Could you check a few things on this model? Use its own coordinates, in mm. A direction names the side the tool comes from. Coordinates: 2 decimals unless noted, no trailing zeros. Loops run counter-clockwise (first coordinate to the right, second up) from the corner with the lowest first, then second, coordinate; pieces in that order, holes last. Notation, with made-up numbers: (84.25, 70.5) - (138.25, 70.5) arc R13 ccw to (138.25, 92.5) - close; hole circle Ø1 at (-27, 45.25). An arc over 180 degrees is marked (long way). Put each result on its own line as item: value. Start each with the question number.
```python
from build123d import *

# Parameters (mm, degrees)
SKETCH1_W                                      = 193.929
SKETCH1_H                                      = 117.602
BOSS_EXTRUDE1_DEPTH                            = 2.667
CUT_EXTRUDE1_DEPTH                             = 0.254
BOSS_EXTRUDE2_DEPTH                            = 0.254
BOSS_EXTRUDE3_DEPTH                            = 1.6002
BOSS_EXTRUDE4_DEPTH                            = 1.6002
BOSS_EXTRUDE5_DEPTH                            = 1.6002
BOSS_EXTRUDE6_DEPTH                            = 1.6002
BOSS_EXTRUDE7_DEPTH                            = 1.6002
SKETCH9_W                                      = 3.683
SKETCH9_H                                      = 3.175
SKETCH10_W                                     = 3.683
SKETCH10_H                                     = 3.175
SKETCH11_W                                     = 3.683
SKETCH11_H                                     = 3.175
SKETCH12_W                                     = 3.683
SKETCH12_H                                     = 3.175
CSK_FOR_M3_FLAT_HEAD_MACHINE_SCREW1_AT_2_COUNT = 2
CSK_FOR_M3_FLAT_HEAD_MACHINE_SCREW1_AT_2_PITCH = 202.702821766
CSK_FOR_M3_FLAT_HEAD_MACHINE_SCREW1_AT_3_COUNT = 2
CSK_FOR_M3_FLAT_HEAD_MACHINE_SCREW1_AT_3_PITCH = 176.276
CSK_FOR_M3_FLAT_HEAD_MACHINE_SCREW1_AT_4_COUNT = 2
CSK_FOR_M3_FLAT_HEAD_MACHINE_SCREW1_AT_4_PITCH = 100.076
FILLET1_R                                      = 5.1562
FILLET2_R                                      = 1.5748
FILLET3_R                                      = 3.9624
FILLET4_R                                      = 4.7498
SKETCH16_W                                     = 24.727732192
SKETCH16_H                                     = 24.727732192
BOSS_EXTRUDE8_DEPTH                            = 40
SKETCH18_W                                     = 40
SKETCH18_H                                     = 40
SKETCH18_W_2                                   = 24.727732192
SKETCH18_H_2                                   = 24.727732192
BOSS_EXTRUDE9_DEPTH                            = 3
CUT_EXTRUDE2_DEPTH                             = 40
CUT_EXTRUDE2_DEPTH_BACK                        = 40
SKETCH17_R                                     = 2
SKETCH19_R                                     = 2
CUT_EXTRUDE3_DEPTH                             = 10
SKETCH20_W                                     = 226.645594452
SKETCH20_H                                     = 139.264160446
SKETCH20_W_2                                   = 98.304113256
SKETCH20_H_2                                   = 70.390599616
CUT_EXTRUDE4_DEPTH                             = 121.248375711
SKETCH21_W                                     = 98.304113256
SKETCH21_H                                     = 2.667
CUT_EXTRUDE5_DEPTH                             = 100.458365049
SKETCH23_R                                     = 2
CUT_EXTRUDE6_DEPTH                             = 49.989794856


with BuildPart() as part:
    # Sketch1 → Boss-Extrude1 (new body)
    with BuildSketch(Plane.XZ.offset(2.667)):
        Rectangle(SKETCH1_W, SKETCH1_H)
    extrude(amount=-BOSS_EXTRUDE1_DEPTH)

    # Sketch2 → Cut-Extrude1 (cut)
    with BuildSketch(Plane.XZ.offset(2.667)):
        Polygon((-74.4728, 55.3085), (-93.472, 36.2712), (-93.472, -36.2712), (-74.4728, -55.3085), (74.4728, -55.3085), (93.472, -36.2712), (93.472, 36.2712), (74.4728, 55.3085), align=None)
    extrude(amount=-CUT_EXTRUDE1_DEPTH, mode=Mode.SUBTRACT)

    # Sketch3 → Boss-Extrude2 (add)
    with BuildSketch(Plane.XZ.offset(2.413)):
        Polygon((92.6846, 35.945510163), (92.6846, -35.945510163), (74.146186127, -54.5211), (-74.146186127, -54.5211), (-92.6846, -35.945510163), (-92.6846, 35.945510163), (-74.146186127, 54.5211), (74.146186127, 54.5211), align=None)
    extrude(amount=BOSS_EXTRUDE2_DEPTH)

    # Sketch4 → Boss-Extrude3 (add)
    with BuildSketch(Plane(origin=(0, 0, 0), x_dir=(-1, 0, 0), z_dir=(0, 1, 0))):
        with BuildLine():
            Line((92.6211, -49.3395), (92.6211, 49.3395))
            ThreePointArc((92.6211, 49.3395), (93.4212, 50.1396), (94.2213, 49.3395))
            Line((94.2213, 49.3395), (94.2213, -49.3395))
            ThreePointArc((94.2213, -49.3395), (93.4212, -50.1396), (92.6211, -49.3395))
        make_face()
    extrude(amount=BOSS_EXTRUDE3_DEPTH)

    # Sketch5 → Boss-Extrude4 (add)
    with BuildSketch(Plane(origin=(0, 0, 0), x_dir=(-1, 0, 0), z_dir=(0, 1, 0))):
        with BuildLine():
            Line((-94.2213, -49.3395), (-94.2213, 49.3395))
            ThreePointArc((-94.2213, 49.3395), (-93.4212, 50.1396), (-92.6211, 49.3395))
            Line((-92.6211, 49.3395), (-92.6211, -49.3395))
            ThreePointArc((-92.6211, -49.3395), (-93.4212, -50.1396), (-94.2213, -49.3395))
        make_face()
    extrude(amount=BOSS_EXTRUDE4_DEPTH)

    # Sketch6 → Boss-Extrude5 (add)
    with BuildSketch(Plane(origin=(0, 0, 0), x_dir=(-1, 0, 0), z_dir=(0, 1, 0))):
        with BuildLine():
            Line((10.4013, -54.4576), (87.5919, -54.4576))
            ThreePointArc((87.5919, -54.4576), (88.392, -55.2577), (87.5919, -56.0578))
            Line((87.5919, -56.0578), (10.4013, -56.0578))
            ThreePointArc((10.4013, -56.0578), (9.6012, -55.2577), (10.4013, -54.4576))
        make_face()
    extrude(amount=BOSS_EXTRUDE5_DEPTH)

    # Sketch7 → Boss-Extrude6 (add)
    with BuildSketch(Plane(origin=(0, 0, 0), x_dir=(-1, 0, 0), z_dir=(0, 1, 0))):
        with BuildLine():
            Line((-87.5919, 56.0578), (87.5919, 56.0578))
            ThreePointArc((87.5919, 56.0578), (88.392, 55.2577), (87.5919, 54.4576))
            Line((87.5919, 54.4576), (-87.5919, 54.4576))
            ThreePointArc((-87.5919, 54.4576), (-88.392, 55.2577), (-87.5919, 56.0578))
        make_face()
    extrude(amount=BOSS_EXTRUDE6_DEPTH)

    # Sketch8 → Boss-Extrude7 (add)
    with BuildSketch(Plane(origin=(0, 0, 0), x_dir=(-1, 0, 0), z_dir=(0, 1, 0))):
        with BuildLine():
            Line((-87.5919, -54.4576), (-10.4013, -54.4576))
            ThreePointArc((-10.4013, -54.4576), (-9.6012, -55.2577), (-10.4013, -56.0578))
            Line((-10.4013, -56.0578), (-87.5919, -56.0578))
            ThreePointArc((-87.5919, -56.0578), (-88.392, -55.2577), (-87.5919, -54.4576))
        make_face()
    extrude(amount=BOSS_EXTRUDE7_DEPTH)

    # Sketch9 → Revolve1 (revolve)
    with BuildSketch(Plane.XY.offset(-50.038), mode=Mode.PRIVATE) as revolve1_sk:
        with Locations((-86.2965, 1.5875)):
            Rectangle(SKETCH9_W, SKETCH9_H)
    revolve(revolve1_sk.sketch.rotate(Axis((-88.138, 3.175, -50.038), (0, -1, 0)), 270), axis=Axis((-88.138, 3.175, -50.038), (0, -1, 0)))

    # Sketch10 → Revolve2 (revolve)
    with BuildSketch(Plane.XY.offset(50.038), mode=Mode.PRIVATE) as revolve2_sk:
        with Locations((89.9795, 1.5875)):
            Rectangle(SKETCH10_W, SKETCH10_H)
    revolve(revolve2_sk.sketch.rotate(Axis((88.138, 3.175, 50.038), (0, -1, 0)), 270), axis=Axis((88.138, 3.175, 50.038), (0, -1, 0)))

    # Sketch11 → Revolve3 (revolve)
    with BuildSketch(Plane.XY.offset(50.038), mode=Mode.PRIVATE) as revolve3_sk:
        with Locations((-86.2965, 1.5875)):
            Rectangle(SKETCH11_W, SKETCH11_H)
    revolve(revolve3_sk.sketch.rotate(Axis((-88.138, 3.175, 50.038), (0, -1, 0)), 270), axis=Axis((-88.138, 3.175, 50.038), (0, -1, 0)))

    # Sketch12 → Revolve4 (revolve)
    with BuildSketch(Plane.XY.offset(-50.038), mode=Mode.PRIVATE) as revolve4_sk:
        with Locations((89.9795, 1.5875)):
            Rectangle(SKETCH12_W, SKETCH12_H)
    revolve(revolve4_sk.sketch.rotate(Axis((88.138, 3.175, -50.038), (0, -1, 0)), 270), axis=Axis((88.138, 3.175, -50.038), (0, -1, 0)))

    # Sketch13 → CSK for M3 Flat Head Machine Screw1 (revolve, cut)
    with BuildSketch(Plane(origin=(88.138, -2.667, -50.038), x_dir=(0, 0, -1), z_dir=(1, 0, 0))):
        Polygon((0, 0), (0, 5.842), (1.6256, 5.842), (1.6256, 3.175), (3.048, 1.538715978), (3.048, 0), align=None)
    csk_for_m3_flat_head_machine_screw1 = revolve(axis=Axis((88.138, -9.017, -50.038), (0, 1, 0)), mode=Mode.SUBTRACT)

    # CSK for M3 Flat Head Machine Screw1 at 2: CSK for M3 Flat Head Machine Screw1 ×2
    with Locations(*[Vector(-0.8696277558645717, 0, 0.4937079766723937) * (i * CSK_FOR_M3_FLAT_HEAD_MACHINE_SCREW1_AT_2_PITCH) for i in range(1, CSK_FOR_M3_FLAT_HEAD_MACHINE_SCREW1_AT_2_COUNT)]):
        add(csk_for_m3_flat_head_machine_screw1, mode=Mode.SUBTRACT)

    # CSK for M3 Flat Head Machine Screw1 at 3: CSK for M3 Flat Head Machine Screw1 ×2
    with Locations(*[(-i * CSK_FOR_M3_FLAT_HEAD_MACHINE_SCREW1_AT_3_PITCH, 0, 0) for i in range(1, CSK_FOR_M3_FLAT_HEAD_MACHINE_SCREW1_AT_3_COUNT)]):
        add(csk_for_m3_flat_head_machine_screw1, mode=Mode.SUBTRACT)

    # CSK for M3 Flat Head Machine Screw1 at 4: CSK for M3 Flat Head Machine Screw1 ×2
    with Locations(*[(0, 0, i * CSK_FOR_M3_FLAT_HEAD_MACHINE_SCREW1_AT_4_PITCH) for i in range(1, CSK_FOR_M3_FLAT_HEAD_MACHINE_SCREW1_AT_4_COUNT)]):
        add(csk_for_m3_flat_head_machine_screw1, mode=Mode.SUBTRACT)

    # Fillet1
    fillet1_edges = [part.edges().sort_by_distance(p)[0] for p in [
        (-96.9645, -1.3335, 58.801),
        (96.9645, -1.3335, 58.801),
        (96.9645, -1.3335, -58.801),
        (-96.9645, -1.3335, -58.801),
    ]]
    fillet(fillet1_edges, radius=FILLET1_R)

    # Fillet2
    fillet2_edges = [part.edges().sort_by_distance(p)[0] for p in [
        (0, -2.667, 58.801),
        (-96.9645, -2.667, 0),
        (0, -2.667, -58.801),
        (96.9645, -2.667, 0),
        (95.454283985, -2.667, -57.290783985),
        (95.454283985, -2.667, 57.290783985),
        (-95.454283985, -2.667, -57.290783985),
        (-95.454283985, -2.667, 57.290783985),
    ]]
    fillet(fillet2_edges, radius=FILLET2_R)

    # Fillet3
    fillet3_edges = [part.edges().sort_by_distance(p)[0] for p in [
        (92.6846, -2.54, 35.945510163),
        (74.146186127, -2.54, 54.5211),
        (-74.146186127, -2.54, 54.5211),
        (-92.6846, -2.54, 35.945510163),
        (-92.6846, -2.54, -35.945510163),
        (-74.146186127, -2.54, -54.5211),
        (74.146186127, -2.54, -54.5211),
        (92.6846, -2.54, -35.945510163),
    ]]
    fillet(fillet3_edges, radius=FILLET3_R)

    # Fillet4
    fillet4_edges = [part.edges().sort_by_distance(p)[0] for p in [
        (-74.4728, -2.54, 55.3085),
        (74.4728, -2.54, 55.3085),
        (93.472, -2.54, 36.2712),
        (93.472, -2.54, -36.2712),
        (74.4728, -2.54, -55.3085),
        (-74.4728, -2.54, -55.3085),
        (-93.472, -2.54, -36.2712),
        (-93.472, -2.54, 36.2712),
    ]]
    fillet(fillet4_edges, radius=FILLET4_R)

    # Sketch16 → Boss-Extrude8 (add)
    with BuildSketch(Plane.XZ.offset(2.667)):
        Rectangle(SKETCH16_W, SKETCH16_H)
    extrude(amount=BOSS_EXTRUDE8_DEPTH)

    # Sketch18 → Boss-Extrude9 (add)
    with BuildSketch(Plane.XZ.offset(2.667)):
        Rectangle(SKETCH18_W, SKETCH18_H)
        Rectangle(SKETCH18_W_2, SKETCH18_H_2, mode=Mode.SUBTRACT)
    extrude(amount=BOSS_EXTRUDE9_DEPTH)

    # Sketch17 → Cut-Extrude2 (cut, two sides: drawn at the far end of the back side and taken through both)
    with BuildSketch(Plane.XZ.offset(2.667).offset(-CUT_EXTRUDE2_DEPTH_BACK)):
        with Locations(Location((-16.181933048, 0, 0), (0, 0, 270))):
            Circle(SKETCH17_R)
        with Locations(Location((0, 16.181933048, 0), (0, 0, 270))):
            Circle(SKETCH17_R)
        with Locations(Location((16.181933048, 0, 0), (0, 0, 270))):
            Circle(SKETCH17_R)
        with Locations(Location((0, -16.181933048, 0), (0, 0, 270))):
            Circle(SKETCH17_R)
    extrude(amount=CUT_EXTRUDE2_DEPTH + CUT_EXTRUDE2_DEPTH_BACK, mode=Mode.SUBTRACT)

    # Sketch19 → Cut-Extrude3 (cut)
    with BuildSketch(Plane.XZ.offset(42.667)):
        with Locations(Location((0, 0, 0), (0, 0, 270))):
            Circle(SKETCH19_R)
    extrude(amount=-CUT_EXTRUDE3_DEPTH, mode=Mode.SUBTRACT)

    # Sketch20 → Cut-Extrude4 (cut, through all)
    with BuildSketch(Plane.XZ.offset(2.667)):
        with Locations((4.399412476, -0.910223271)):
            Rectangle(SKETCH20_W, SKETCH20_H)
        with Locations((-6.674970653, -1.97215042)):
            Rectangle(SKETCH20_W_2, SKETCH20_H_2, mode=Mode.SUBTRACT)
    extrude(amount=-CUT_EXTRUDE4_DEPTH, mode=Mode.SUBTRACT)

    # Sketch21 → Cut-Extrude5 (cut, through all)
    with BuildSketch(Plane(origin=(0, 0, -37.167450228), x_dir=(-1, 0, 0), z_dir=(0, 0, -1))):
        with Locations((6.674970653, -1.3335)):
            Rectangle(SKETCH21_W, SKETCH21_H)
    extrude(amount=-CUT_EXTRUDE5_DEPTH, mode=Mode.SUBTRACT)

    # Sketch23 → Cut-Extrude6 (cut, through all)
    with BuildSketch(Plane.XZ.offset(42.667)):
        with Locations(Location((7.181933048, 0, 0), (0, 0, 270))):
            Circle(SKETCH23_R)
        with Locations(Location((0, 7.181933048, 0), (0, 0, 90))):
            Circle(SKETCH23_R)
    extrude(amount=-CUT_EXTRUDE6_DEPTH, mode=Mode.SUBTRACT)


solid = part.part
```
(1) Which directions (+Z, -Z, +X, -X, +Y, -Y) give clear straight access to the entire face, cutting with the end or side of a thin tool? Please do faces 1 (the flat face through (0, -24, 12.364)), 2 (the flat face through (0, -24, -12.364)), 3 (the flat face through (-20, -4, 0)), 4 (the flat face through (12.364, -24, 0)), 5 (the cylindrical face through (-2, -38, 0)).
(2) If we mould it in two halves opening along Z, with no side actions, what happens to faces 6 (the flat face through (0, -4, 20)), 7 (the flat face through (0, -32.667, 0)), 8 (the flat face through (-12.364, -24, 0))? For each: pulls with the +Z half, pulls with the -Z half, needs draft (parallel to the pull), parting line crosses it, or undercut.
(3) I want a section at A-A on z = 0. List the corners of the cut face in (x, y) for me, and give its area (3 significant figures).
(4) For pin 1 Ø8 at (y, z) = (-31.5, 7.5) entering from +X; pin 2 Ø4.5 at (x, z) = (16.18, 0) entering from -Y; pin 3 Ø7.5 at (x, y) = (-1, -22) entering from -Z, each with a flat end and sliding along its axis, tell me the tip position at first contact or that it passes through.
(5) I want a section at C-C on x = 4. List the corners of the cut face in (y, z) for me, and give its area (3 significant figures).
(6) I need wall thicknesses on L1, parallel to X at y = -35, z = 0; L2, parallel to X at y = -3, z = 0; L3, parallel to X at y = -21, z = 0. Which ranges of each line are inside material? Lowest first, please. Write a range as [from, to].
(7) I want a section at B-B on x = 0. List the corners of the cut face in (y, z) for me.
(8) I want a section at D-D on z = -11. List the corners of the cut face in (x, y) for me.
Answer sheet:
1. face 1: +Z, +X, -X, -Y
1. face 2: -Z, +X, -X, -Y
1. face 3: +Z, -Z, -X, +Y, -Y
1. face 4: +Z, -Z, +X, -Y
1. face 5: -Y
2. face 6: pulls with the +Z half
2. face 7: undercut
2. face 8: needs draft
3. outline: (-20, -5.67) - (-18.18, -5.67) - (-18.18, -2.67) - (-20, -2.67) - close; (-14.18, -5.67) - (-12.36, -5.67) - (-12.36, -42.67) - (-2, -42.67) - (-2, -32.67) - (2, -32.67) - (2, -42.67) - (5.18, -42.67) - (5.18, -2.67) - (-14.18, -2.67) - close; (9.18, -42.67) - (12.36, -42.67) - (12.36, -5.67) - (14.18, -5.67) - (14.18, -2.67) - (9.18, -2.67) - close; (18.18, -5.67) - (20, -5.67) - (20, -2.67) - (18.18, -2.67) - close
3. area: 811 mm^2
4. pin 1: stops at x = 12.36
4. pin 2: stops at y = -5.67
4. pin 3: stops at z = -12.36
5. outline: (-42.67, -12.36) - (-5.67, -12.36) - (-5.67, -20) - (-2.67, -20) - (-2.67, 20) - (-5.67, 20) - (-5.67, 12.36) - (-42.67, 12.36) - close
5. area: 1,030 mm^2
6. L1: x = [-12.36, -2], [2, 5.18], [9.18, 12.36]
6. L2: x = [-20, -18.18], [-14.18, 5.18], [9.18, 14.18], [18.18, 20]
6. L3: x = [-12.36, 5.18], [9.18, 12.36]
7. outline: (-42.67, -12.36) - (-5.67, -12.36) - (-5.67, -14.18) - (-2.67, -14.18) - (-2.67, 5.18) - (-42.67, 5.18) - (-42.67, 2) - (-32.67, 2) - (-32.67, -2) - (-42.67, -2) - close; (-42.67, 9.18) - (-2.67, 9.18) - (-2.67, 14.18) - (-5.67, 14.18) - (-5.67, 12.36) - (-42.67, 12.36) - close; (-5.67, -20) - (-2.67, -20) - (-2.67, -18.18) - (-5.67, -18.18) - close; (-5.67, 18.18) - (-2.67, 18.18) - (-2.67, 20) - (-5.67, 20) - close
8. outline: (-20, -5.67) - (-12.36, -5.67) - (-12.36, -42.67) - (12.36, -42.67) - (12.36, -5.67) - (20, -5.67) - (20, -2.67) - (-20, -2.67) - close
